Input: part model. Units: mm. Frame: model coordinates. A direction names the side the tool comes from. Give positions to 0.01 mm unless a question says otherwise; leave off trailing zeros. Order: outer loops, then holes, each group sorted by start corner. A loop starts at its lowest first (then second) coordinate and runs counter-clockwise, first axis right, second up. Notation, with made-up numbers: (75.25, 75.5) - (128.25, 75.5) arc R21 ccw to (128.25, 102.5) - close; hole circle Ø2 at (25.5, 75). An arc over 180 degrees is marked (long way). Answer in a Markdown table with one row per item. Add a question column.
1. Section query B-B on z = 3. Return loops of the section in (x, y) (3 decimals), and give its area (3 significant figures).
2. Section query A-A on x = 66.04. Return loops of the section in (y, z).
3. Ray query, line 1 (X direction, y = 0.4, z = 4.5) (3 decimals); line 2 (X direction, y = 1.95, z = 0) (1 decimal); line 3 (X direction, y = 1.25, z = 6.5) (3 decimals). Return the intervals inside material, ascending. Write a range as [from, to].
4. Contact query for flat-ended pins moving along their axis: pin 1 (1.8 mm diameter, centred on x = 33.02, z = 3.175, fed in from -Y); pin 2 (1.3 mm diameter, centred on x = 51, y = 1.5, fed in from -Z); pin 3 (0.8 mm diameter, centred on x = 47, y = 2, fed in from +Z); pin 4 (1 mm diameter, centred on x = 11.5, y = 2, fed in from -Z). Output: stop coordinate, or through.
5. Access query for faces 4 (the face through (52, 1, 0.254)), 5 (the face through (49, 1, 10.414)), 6 (the face through (67.614, 1.252, 2.968)), 7 (the face through (31.52, 1, 4)). Directions: +Z, -Z, +X, -X, +Y, -Y. A direction counts if a zero-diameter tool reaches every point of the face in a straight line with its end or side. Return the directions, or none.
6. Section query C-C on y = 1.2. Return loops of the section in (x, z) (1 decimal).
7. Mould query, pull axis Z, two halves, no side actions, for faces 1 (the face through (-0.966, 1.252, -1.26)), 2 (the face through (10.74, 1.25, -2.13)), 3 (the face through (29.76, 1.25, 12.71)). Classes: released by +Z, released by -Z, zero draft, split by the parting line, or undercut.
8. Section query D-D on x = 33.02. Return loops of the section in (y, z), and give its area (3 significant figures).
```python
from build123d import *

# Parameters (mm, degrees)
SKETCH1_R           = 1.016
SKETCH1_R_2         = 1.5875
SKETCH1_R_3         = 1.0922
BOSS_EXTRUDE1_DEPTH = 2.54
SKETCH2_W           = 13.662102681
SKETCH2_H           = 9.772536082
CUT_EXTRUDE1_DEPTH  = 2.54


with BuildPart() as part:
    # Sketch1 → Boss-Extrude1 (new body)
    with BuildSketch(Plane(origin=(0, 0, 0), x_dir=(1, 0, 0), z_dir=(0, 1, 0))):
        Polygon((-3.175, 3.429), (-3.175, -10.414), (4.467211682, -14.946323026), (23.497546316, -14.946323026), (36.195, -10.414), (62.473953038, -10.414), (71.12, -6.112857804), (71.12, -0.254), (24.145875, -0.254), (3.429, 3.429), align=None)
        with Locations(Location((33.02, -3.175, 0), (0, 0, 270))):
            Circle(SKETCH1_R, mode=Mode.SUBTRACT)
        with Locations(Location((66.04, -3.175, 0), (0, 0, 270))):
            Circle(SKETCH1_R_2, mode=Mode.SUBTRACT)
        with Locations(Location((0, 0, 0), (0, 0, 270))):
            Circle(SKETCH1_R_2, mode=Mode.SUBTRACT)
        with Locations(Location((58.296606113, -3.175, 0), (0, 0, 270))):
            Circle(SKETCH1_R_3, mode=Mode.SUBTRACT)
    extrude(amount=BOSS_EXTRUDE1_DEPTH)

    # Sketch2 → Cut-Extrude1 (cut)
    with BuildSketch(Plane.XZ):
        with Locations((24.68894866, 3.393977835)):
            Rectangle(SKETCH2_W, SKETCH2_H)
    extrude(amount=-CUT_EXTRUDE1_DEPTH, mode=Mode.SUBTRACT)


solid = part.part
```
Answer:
| question | item | result |
|---|---|---|
| 1 | outline | (-3.175, 0) - (17.858, 0) - (17.858, 2.54) - (-3.175, 2.54) - close; (31.52, 0) - (32.019, 0) - (32.019, 2.54) - (31.52, 2.54) - close; (34.021, 0) - (57.219, 0) - (57.219, 2.54) - (34.021, 2.54) - close; (59.375, 0) - (64.462, 0) - (64.462, 2.54) - (59.375, 2.54) - close; (67.618, 0) - (71.12, 0) - (71.12, 2.54) - (67.618, 2.54) - close |
| 1 | area | 135 mm² |
| 2 | outline | (0, 0.25) - (2.54, 0.25) - (2.54, 1.59) - (0, 1.59) - close; (0, 4.76) - (2.54, 4.76) - (2.54, 8.64) - (0, 8.64) - close |
| 3 | line 1 | x = [-3.175, 17.858], [31.52, 65.166], [66.914, 71.12] |
| 3 | line 2 | x = [-3.2, -1.6], [1.6, 17.9] |
| 3 | line 3 | x = [-3.175, 17.858], [31.52, 70.342] |
| 4 | pin 1 | passes through |
| 4 | pin 2 | stops at z = 0.25 |
| 4 | pin 3 | stops at z = 10.41 |
| 4 | pin 4 | stops at z = -2.08 |
| 5 | face 4 | -Z, +X, +Y, -Y |
| 5 | face 5 | +Z, +X, +Y, -Y |
| 5 | face 6 | +Y, -Y |
| 5 | face 7 | -Z, +Y, -Y |
| 6 | outline | (-3.2, -3.4) - (3.4, -3.4) - (17.9, -0.9) - (17.9, 8.3) - (31.5, 8.3) - (31.5, 0.3) - (71.1, 0.3) - (71.1, 6.1) - (62.5, 10.4) - (36.2, 10.4) - (23.5, 14.9) - (4.5, 14.9) - (-3.2, 10.4) - close; hole circle Ø3.2 at (0, 0); hole circle Ø2 at (33, 3.2); hole circle Ø2.2 at (58.3, 3.2); hole circle Ø3.2 at (66, 3.2) |
| 7 | face 1 | undercut |
| 7 | face 2 | released by -Z |
| 7 | face 3 | released by +Z |
| 8 | outline | (0, 0.25) - (2.54, 0.25) - (2.54, 2.16) - (0, 2.16) - close; (0, 4.19) - (2.54, 4.19) - (2.54, 11.55) - (0, 11.55) - close |
| 8 | area | 23.5 mm² |
